Work out the finished part from the listing and answer in its coordinate system (mm). Face numbers are marked on the shaded views. Coordinates: 2 decimals unless noted, no trailing zeros. Loops run counter-clockwise (first coordinate to the right, second up) from the corner with the lowest first, then second, coordinate; pieces in that order, holes last. Notation, with made-up numbers: (82, -37.5) -> (86, -37.5) arc R13 ccw to (86, -18.5) -> close; hole circle Ø11 at (38.5, -11.75). An arc over 180 degrees is marked (long way). Answer as CSV lines item,"result".
```python
from build123d import *

# Parameters (mm, degrees)
SKETCH1_R            = 15
BOSS_EXTRUDE1_DEPTH  = 3
SKETCH2_R            = 2.5
CUT_EXTRUDE1_DEPTH   = 3
SKETCH3_R            = 7.5
BOSS_EXTRUDE3_DEPTH  = 3
FILLET1_R            = 5
SKETCH4_R            = 2.917424305
BOSS_EXTRUDE4_DEPTH  = 200
SKETCH5_R            = 4
BOSS_EXTRUDE5_DEPTH  = 2
SKETCH6_R            = 2.5
BOSS_EXTRUDE6_DEPTH  = 2
SKETCH7_R            = 1.5
BOSS_EXTRUDE7_DEPTH  = 100
SKETCH8_R            = 2
BOSS_EXTRUDE9_DEPTH  = 3
FILLET4_R            = 1
SKETCH9_R            = 1
BOSS_EXTRUDE10_DEPTH = 30
SKETCH10_R           = 2.5
BOSS_EXTRUDE11_DEPTH = 1
SKETCH11_R           = 1
BOSS_EXTRUDE12_DEPTH = 2
BOSS_EXTRUDE13_DEPTH = 50


with BuildPart() as part:
    # Sketch1 → Boss-Extrude1 (new body)
    with BuildSketch(Plane(origin=(0, 0, 0), x_dir=(1, 0, 0), z_dir=(0, 1, 0))):
        with Locations(Location((0, 0, 0), (0, 0, 270))):
            Circle(SKETCH1_R)
    extrude(amount=BOSS_EXTRUDE1_DEPTH)

    # Sketch2 → Cut-Extrude1 (cut)
    with BuildSketch(Plane(origin=(0, 3, 0), x_dir=(1, 0, 0), z_dir=(0, 1, 0))):
        with Locations(Location((0, 12, 0), (0, 0, 270))):
            Circle(SKETCH2_R)
        with Locations(Location((12, 0, 0), (0, 0, 270))):
            Circle(SKETCH2_R)
        with Locations(Location((0, -12, 0), (0, 0, 270))):
            Circle(SKETCH2_R)
        with Locations(Location((-12, 0, 0), (0, 0, 270))):
            Circle(SKETCH2_R)
    extrude(amount=-CUT_EXTRUDE1_DEPTH, mode=Mode.SUBTRACT)

    # Sketch3 → Boss-Extrude3 (add)
    with BuildSketch(Plane(origin=(0, 3, 0), x_dir=(1, 0, 0), z_dir=(0, 1, 0))):
        with Locations(Location((0, 0, 0), (0, 0, 270))):
            Circle(SKETCH3_R)
    extrude(amount=BOSS_EXTRUDE3_DEPTH)

    # Fillet1
    # the kernel refuses this fillet: 5 mm, written as the material it takes off along each edge
    with BuildSketch(Plane(origin=(0, 6, 0), x_dir=(0, 0, 1), z_dir=(-1, 0, 0))) as fillet1_piece_1:
        with BuildLine():
            CenterArc((2.917424305, -5), FILLET1_R, 23.578178478, 66.421821522)
            Line((2.917424305, 0), (2.917424305, 0.1))
            Line((2.917424305, 0.1), (7.5, 0.1))
            Line((7.5, 0.1), (7.6, 0))
            ThreePointArc((7.6, 0), (7.6, -1.5), (7.591651514, -2.96))
            Line((7.591651514, -2.96), (7.5, -3))
        make_face()
    revolve(axis=Axis((0, 6, 0), (0, 1, 0)), mode=Mode.SUBTRACT)

    # Sketch4 → Boss-Extrude4 (add)
    with BuildSketch(Plane(origin=(0, 6, 0), x_dir=(1, 0, 0), z_dir=(0, 1, 0))):
        with Locations(Location((0, 0, 0), (0, 0, 270))):
            Circle(SKETCH4_R)
    extrude(amount=BOSS_EXTRUDE4_DEPTH)

    # Sketch5 → Boss-Extrude5 (add)
    with BuildSketch(Plane(origin=(0, 206, 0), x_dir=(1, 0, 0), z_dir=(0, 1, 0))):
        with Locations(Location((0, 0, 0), (0, 0, 270))):
            Circle(SKETCH5_R)
    extrude(amount=BOSS_EXTRUDE5_DEPTH)

    # Sketch6 → Boss-Extrude6 (add)
    with BuildSketch(Plane(origin=(0, 208, 0), x_dir=(1, 0, 0), z_dir=(0, 1, 0))):
        with Locations(Location((0, 0, 0), (0, 0, 270))):
            Circle(SKETCH6_R)
    extrude(amount=BOSS_EXTRUDE6_DEPTH)

    # Sketch7 → Boss-Extrude7 (add)
    with BuildSketch(Plane(origin=(0, 210, 0), x_dir=(1, 0, 0), z_dir=(0, 1, 0))):
        with Locations(Location((0, 0, 0), (0, 0, 270))):
            Circle(SKETCH7_R)
    extrude(amount=BOSS_EXTRUDE7_DEPTH)

    # Sketch8 → Boss-Extrude9 (add)
    with BuildSketch(Plane(origin=(0, 310, 0), x_dir=(1, 0, 0), z_dir=(0, 1, 0))):
        with Locations(Location((0, 0, 0), (0, 0, 270))):
            Circle(SKETCH8_R)
    extrude(amount=BOSS_EXTRUDE9_DEPTH)

    # Fillet4
    # the kernel refuses this fillet: 1 mm, written as the material it takes off along each edge
    with BuildSketch(Plane(origin=(0, 310, 0), x_dir=(0, 0, 1), z_dir=(-1, 0, 0))) as fillet4_piece_1:
        with BuildLine():
            CenterArc((1, 0.866025404), FILLET4_R, 300, 60)
            Line((1.5, 0), (1.51, -0.017320508))
            ThreePointArc((1.51, -0.017320508), (1.75, -0.02), (2, -0.02))
            Line((2, -0.02), (2.02, 0))
            Line((2.02, 0), (2.02, 0.866025404))
            Line((2.02, 0.866025404), (2, 0.866025404))
        make_face()
    revolve(axis=Axis((0, 310, 0), (0, 1, 0)), mode=Mode.SUBTRACT)
    with BuildSketch(Plane(origin=(0, 313, 0), x_dir=(0, 0, 1), z_dir=(-1, 0, 0))) as fillet4_piece_2:
        with BuildLine():
            CenterArc((2 - FILLET4_R, -FILLET4_R), FILLET4_R, 0, 90)
            Line((2 - FILLET4_R, 0), (2 - FILLET4_R, FILLET4_R * 0.02))
            Line((2 - FILLET4_R, FILLET4_R * 0.02), (2 + FILLET4_R * 0.02, FILLET4_R * 0.02))
            Line((2 + FILLET4_R * 0.02, FILLET4_R * 0.02), (2 + FILLET4_R * 0.02, -FILLET4_R))
            Line((2 + FILLET4_R * 0.02, -FILLET4_R), (2, -FILLET4_R))
        make_face()
    revolve(axis=Axis((0, 313, 0), (0, 1, 0)), mode=Mode.SUBTRACT)

    # Sketch9 → Boss-Extrude10 (add)
    with BuildSketch(Plane(origin=(0, 313, 0), x_dir=(1, 0, 0), z_dir=(0, 1, 0))):
        with Locations(Location((0, 0, 0), (0, 0, 270))):
            Circle(SKETCH9_R)
    extrude(amount=BOSS_EXTRUDE10_DEPTH)

    # Sketch10 → Boss-Extrude11 (add)
    with BuildSketch(Plane(origin=(0, 343, 0), x_dir=(1, 0, 0), z_dir=(0, 1, 0))):
        with Locations(Location((0, 0, 0), (0, 0, 270))):
            Circle(SKETCH10_R)
    extrude(amount=BOSS_EXTRUDE11_DEPTH)

    # Sketch11 → Boss-Extrude12 (add)
    with BuildSketch(Plane(origin=(0, 344, 0), x_dir=(1, 0, 0), z_dir=(0, 1, 0))):
        with Locations(Location((0, 0, 0), (0, 0, 270))):
            Circle(SKETCH11_R)
    extrude(amount=BOSS_EXTRUDE12_DEPTH)

    # Sketch12 → Boss-Extrude13 (add)
    with BuildSketch(Plane.XZ):
        with BuildLine():
            Line((0, 15), (0, 15.5))
            ThreePointArc((0, 15.5), (-15.5, 0), (0, -15.5))
            Line((0, -15.5), (0, -15))
            ThreePointArc((0, -15), (-15, 0), (0, 15))
        make_face()
    extrude(amount=-BOSS_EXTRUDE13_DEPTH)


solid = part.part
```
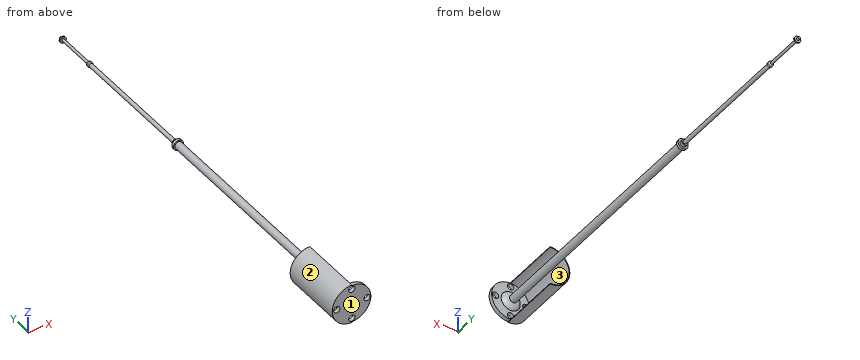
(1) Consider line 1 along X through (y, z) = (2.35, 0); line 2 along Y through (x, z) = (12.5, -4); line 3 along Z through (x, y) = (0.5, 89.5). Determine where each line is inside the solid, lowest interval first.
Computed values:
line 1,"-15.5 to -14.5, -9.5 to 9.5, 14.5 to 15"
line 2,"0 to 3"
line 3,"-2.87 to 2.87"
(2) A cutting plane is placed at A-A, the plane y = 42. Write down the section's boundary in (x, z).
Computed values:
outline,"circle Ø5.83 at (0, 0); (0, -15.5) -> (0, -15) arc R15 cw to (0, 15) -> (0, 15.5) arc R15.5 ccw to start"
(3) For a pull along X with two mould halves and no side action, classify the marked faces 1, 2 and 3 as pulls with the +X half, pulls with the -X half, needs draft (parallel to the pull), parting line crosses it, or undercut.
Computed values:
face 1,"needs draft"
face 2,"pulls with the -X half"
face 3,"undercut"
(4) Flat-ended cylindrical pins translate along their axes: pin 1 Ø3 at (y, z) = (43.5, 9.5) entering from -X; pin 2 Ø6.5 at (x, z) = (-1.5, -1.5) entering from +Y; pin 3 Ø8 at (x, y) = (3, 224) entering from +Z; pin 4 Ø5 at (y, z) = (128, -2) entering from -X. Find the tip coordinate at first contact, or state that the pin passes through.
Computed values:
pin 1,"x = -13.28"
pin 2,"y = 346"
pin 3,"z = 1.5"
pin 4,"x = -2.92"
